from build123d import *

# Parameters (mm, degrees)
SKETCH2_W           = 24.892
SKETCH2_H           = 22.86
BOSS_EXTRUDE1_DEPTH = 3.175
SKETCH3_W           = 2.54
SKETCH3_H           = 10.16
BOSS_EXTRUDE2_DEPTH = 6.35
SKETCH4_W           = 24.892
SKETCH4_H           = 3.175
BOSS_EXTRUDE3_DEPTH = 6.35


with BuildPart() as part:
    # Sketch2 → Boss-Extrude1 (new body)
    with BuildSketch(Plane(origin=(0, 0, 0), x_dir=(1, 0, 0), z_dir=(0, 1, 0))):
        Rectangle(SKETCH2_W, SKETCH2_H)
    extrude(amount=BOSS_EXTRUDE1_DEPTH)

    # Sketch3 → Boss-Extrude2 (add)
    with BuildSketch(Plane(origin=(0, 3.175, 0), x_dir=(1, 0, 0), z_dir=(0, 1, 0))):
        with Locations((11.176, -6.35)):
            Rectangle(SKETCH3_W, SKETCH3_H)
        with Locations((-11.176, -6.35)):
            Rectangle(SKETCH3_W, SKETCH3_H)
    extrude(amount=BOSS_EXTRUDE2_DEPTH)

    # Sketch4 → Boss-Extrude3 (add)
    with BuildSketch(Plane.XZ):
        with Locations((0, -9.8425)):
            Rectangle(SKETCH4_W, SKETCH4_H)
    extrude(amount=BOSS_EXTRUDE3_DEPTH)


solid = part.part
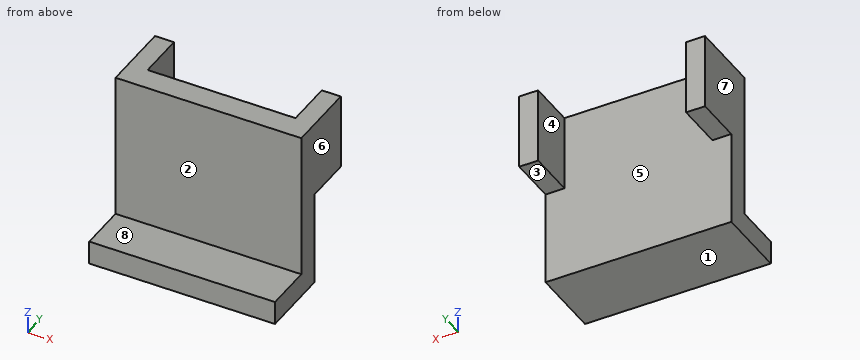
Work out the finished part from the listing and answer in its coordinate system (mm). Face numbers are marked on the shaded views. A direction names the side the tool comes from. Coordinates: 2 decimals unless noted, no trailing zeros. Write each loop counter-clockwise with the first axis right and the second up, starting at its lowest first coordinate (ties: lowest second). Pieces come first, ordered by that corner, then holes. Notation, with made-up numbers: M 57,1 L 63,1 A21 ccw 63,34 Z; hole C 31.25,-11.5 d10. An arc over 180 degrees is marked long. Write item = value, one per line.
1. For the marked faces 1, 2, 3 and 4, determine the directions among +Z, -Z, +X, -X, +Y, -Y from which every point of the face is accessible in a straight line to the end or side of a thin tool.
Solution:
face_1 = -Z, +X, -X, +Y, -Y
face_2 = +Z, +X, -X, -Y
face_3 = -Z, +X, -X, +Y
face_4 = +Z, -Z, +Y
2. Determine the mould class of the marked faces 5, 6, 7 and 8 for opening direction X: released by +X, released by -X, zero draft, split by the parting line, or undercut.
Solution:
face_5 = undercut
face_6 = released by +X
face_7 = released by -X
face_8 = zero draft
3. Flat-ended cylindrical pins translate along their axes: pin 1 (1 mm diameter, centred on x = -5, z = -5, fed in from +Y) (3 decimals); pin 2 (0.8 mm diameter, centred on x = -10.5, y = 5.5, fed in from -Z); pin 3 (3 mm diameter, centred on x = -2, y = -4, fed in from +Z) (3 decimals). Find the tip coordinate at first contact, or state that the pin passes through.
Solution:
pin_1 = 3.175
pin_2 = 1.27
pin_3 = -8.255
4. The part is cut by section B-B (z = 5). Determine the outline of the cut face in (x, y) (3 decimals).
Solution:
outline = M -12.446,0 L 12.446,0 L 12.446,9.525 L 9.906,9.525 L 9.906,3.175 L -9.906,3.175 L -9.906,9.525 L -12.446,9.525 Z
5. The part is cut by section C-C (x = -5.25). Determine the outline of the cut face in (y, z) (3 decimals), then the cut area to 3 significant figures.
Solution:
outline = M -6.35,-11.43 L 3.175,-11.43 L 3.175,11.43 L 0,11.43 L 0,-8.255 L -6.35,-8.255 Z
area = 92.7 mm2
6. The part is cut by section D-D (y = -1). Determine the outline of the cut face in (x, z) (3 decimals).
Solution:
outline = M -12.446,-11.43 L 12.446,-11.43 L 12.446,-8.255 L -12.446,-8.255 Z
7. The part is cut by section A-A (y = 7.25). Determine the outline of the cut face in (x, z), then the cut area to 3 significant figures.
Solution:
outline = M -12.45,1.27 L -9.91,1.27 L -9.91,11.43 L -12.45,11.43 Z; M 9.91,1.27 L 12.45,1.27 L 12.45,11.43 L 9.91,11.43 Z
area = 51.6 mm2
8. Straight lines are drawn through the part: line 1 (X direction, y = 7, z = 10.25); line 2 (Y direction, x = 3, z = 1.25) (3 decimals); line 3 (Z direction, x = 0, y = -0.25) (3 decimals). For each, find the intervals that lie inside material, in ascending order. Write a range as from..to.
Solution:
line_1 = -12.45..-9.91, 9.91..12.45
line_2 = 0..3.175
line_3 = -11.43..-8.255
